Check sheet for the drawn part. Datum: minimum x, y, z corner. Units: mm. A direction names the side the tool comes from. Give positions to 0.01 mm unless a question says otherwise; leave off trailing zeros. Loops run counter-clockwise (first coordinate to the right, second up) from the corner with the lowest first, then second, coordinate; pieces in that order, holes last.
1. Release check for a two-part mould opening along Z. For the marked faces 1, 2, 3 and 4 record: +Z half, -Z half, draft (parallel to the pull), parting line (faces both ways), or undercut.
2. Cross-section at A-A, the plane z = 24. Record the cut outline in (x, y).
3. Go/stop test with flat-tipped pins: pin 1 Ø2 at (x, y) = (6.5, 2.5) entering from +Z; pin 2 Ø1.2 at (y, z) = (2, 24.5) entering from -X. Record where each tip stops, or that it passes through.
4. Cross-section at D-D, the plane x = 23.95. Record the cut outline in (y, z).
5. Tool access check on the marked faces 5 and 6. Record the directions out of +Z, -Z, +X, -X, +Y, -Y that give a thin tool (end or side, any length) a straight path to the whole face; none if there is none.
6. Material ranges on L1, parallel to X at y = 3, z = 26; L2, parallel to Z at x = 2.6, y = 1.65; L3, parallel to X at y = 3, z = 6, recorded low to high.
7. Cross-section at C-C, the plane y = 1.8. Record the cut outline in (x, z), plus the area to 3 significant figures.
8. Cross-section at B-B, the plane x = 2.6. Record the cut outline in (y, z).
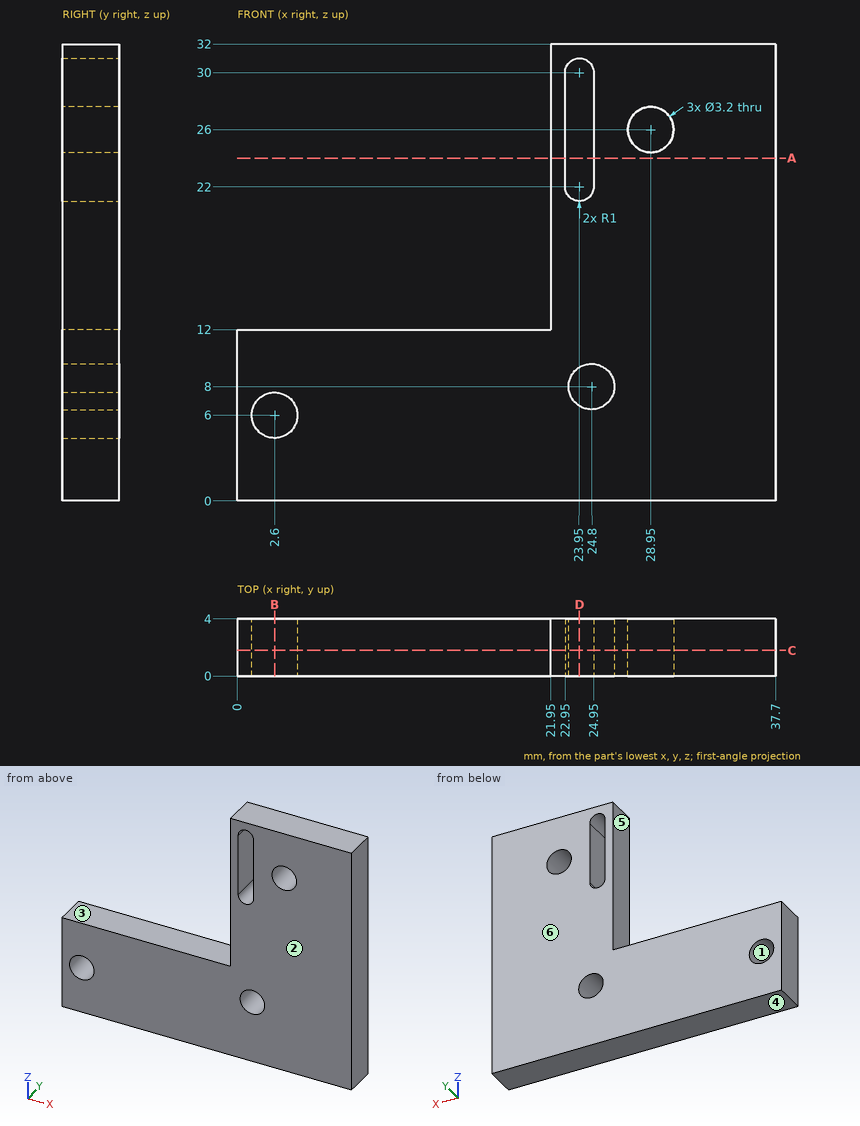
Result:
1. face 1: undercut
1. face 2: draft
1. face 3: +Z half
1. face 4: -Z half
2. outline: (21.95, 0) - (22.95, 0) - (22.95, 4) - (21.95, 4) - close; (24.95, 0) - (37.7, 0) - (37.7, 4) - (24.95, 4) - close
3. pin 1: stops at z = 12
3. pin 2: stops at x = 21.95
4. outline: (0, 0) - (4, 0) - (4, 6.64) - (0, 6.64) - close; (0, 9.36) - (4, 9.36) - (4, 21) - (0, 21) - close; (0, 31) - (4, 31) - (4, 32) - (0, 32) - close
5. face 5: +Z, -X, +Y, -Y
5. face 6: +Z, -Z, +X, -X, +Y
6. L1: x = 21.95 to 22.95, 24.95 to 27.35, 30.55 to 37.7
6. L2: z = 0 to 4.4, 7.6 to 12
6. L3: x = 0 to 1, 4.2 to 37.7
7. outline: (0, 0) - (37.7, 0) - (37.7, 32) - (21.95, 32) - (21.95, 12) - (0, 12) - close; hole circle Ø3.2 at (2.6, 6); hole (22.95, 22) arc R1 ccw to (24.95, 22) - (24.95, 30) arc R1 ccw to (22.95, 30) - close; hole circle Ø3.2 at (24.8, 8); hole circle Ø3.2 at (28.95, 26)
7. area: 724 mm2
8. outline: (0, 0) - (4, 0) - (4, 4.4) - (0, 4.4) - close; (0, 7.6) - (4, 7.6) - (4, 12) - (0, 12) - close
